Geometry check sheet. Reference: the model listing, model coordinates, mm. A direction names the side the tool comes from. Round coordinates to 2 decimals unless told otherwise and drop trailing zeros. Order: outer loops, then holes, each group sorted by start corner. A loop starts at its lowest first (then second) coordinate and runs counter-clockwise, first axis right, second up. Notation, with made-up numbers: (17, 31) -> (75, 31) arc R18 ccw to (75, 49) -> close; hole circle Ø4 at (19.5, 42). An arc over 180 degrees is marked (long way). Use a Markdown table: item, result. Add a question column.
Item 1: Gauge pin test, flat ends, axial feed: pin 1 Ø1 at (x, z) = (284.5, -15.5) entering from -Y; pin 2 Ø1.5 at (x, y) = (129, 3) entering from -Z; pin 3 Ø13 at (y, z) = (3, 1) entering from +X. Record the tip position at first contact, or that the pin passes through.
Item 2: Sectioned sample at A-A, the plane x = 343. Record the cut outline in (y, z), and give its area (3 significant figures).
Item 3: Material ranges on probe 1 along Z at (x, y) = (8.25, 0); probe 2 along Z at (x, y) = (312.5, -2); probe 3 along X at (y, z) = (16, -8.5), recorded low to high. Write a range as [from, to].
Item 4: Mould release check, pull along Y, two halves, no side actions. Record for faces 4 (the cylindrical face through (457.9, -14.18, 1.86)), 5 (the cylindrical face through (8.112, 2.285, 3.584)), 6 (the flat face through (12.4, 13, 0)): pulls with the +Y half, pulls with the -Y half, needs draft (parallel to the pull), parting line crosses it, or undercut.
Item 5: Set-up check for faces 1 (the flat face through (457.5, -11, -10)), 2 (the flat face through (13, -11, 10)), 3 (the cylindrical face through (232.18, -0.97, 22.06)): record each of +Z, -Z, +X, -X, +Y, -Y from which the full face is reachable in a straight line by a thin tool's end or side.
from build123d import *

# Parameters (mm, degrees)
F2_SIZE2 = 0.2309401077
F2_SIZE  = 0.4
F4_D     = 8.5


with BuildPart() as f1:
    # F0 (on Front) → F1 (revolve)
    with BuildSketch(Plane.XZ):
        with BuildLine():
            Line((0, 0), (0, -12.5))
            Line((0, -12.5), (12.4, -12.5))
            Line((12.4, -12.5), (12.4, -14.3))
            Line((12.4, -14.3), (12.8, -14.3))
            ThreePointArc((12.8, -14.3), (12.9414213562, -14.3585786438), (13, -14.5))
            Line((13, -14.5), (13, -23.582))
            ThreePointArc((13, -23.582), (13.4393398282, -24.6426601718), (14.5, -25.082))
            Line((14.5, -25.082), (456, -25.082))
            ThreePointArc((456, -25.082), (457.0606601718, -24.6426601718), (457.5, -23.582))
            Line((457.5, -23.582), (457.5, -14.5))
            ThreePointArc((457.5, -14.5), (457.5585786438, -14.3585786438), (457.7, -14.3))
            Line((457.7, -14.3), (458.1, -14.3))
            Line((458.1, -14.3), (458.1, -12.5))
            Line((458.1, -12.5), (470.5, -12.5))
            Line((470.5, -12.5), (470.5, -10.5))
            Line((470.5, -10.5), (454.5, -10.5))
            Line((454.5, -10.5), (454.5, -22.082))
            Line((454.5, -22.082), (16, -22.082))
            Line((16, -22.082), (16, 0))
            Line((16, 0), (0, 0))
        make_face()
    revolve(axis=Axis((8, 0, 0), (-1, 0, 0)))

    # F2
    f2_edges = [f1.edges().sort_by_distance(p)[0] for p in [
        (0, 0, 12.5),
    ]]
    f2_side = f1.faces().sort_by_distance((6.2, 0, 12.5))[0]
    chamfer(f2_edges, length=F2_SIZE, length2=F2_SIZE2, reference=f2_side)

    # F4 (through all)
    with Locations(Plane(origin=(0, 0, 0), x_dir=(0, -1, 0), z_dir=(-1, 0, 0))):
        with Locations((0, 0)):
            Hole(F4_D / 2)


solid = f1.part
Found:
| question | item | result |
|---|---|---|
| 1 | pin 1 | stops at y = -20.1 |
| 1 | pin 2 | stops at z = -24.98 |
| 1 | pin 3 | stops at x = 16 |
| 2 | outline | circle Ø50.16 at (0, 0); hole circle Ø44.16 at (0, 0) |
| 2 | area | 445 mm2 |
| 3 | probe 1 | z = [-12.5, -4.25], [4.25, 12.5] |
| 3 | probe 2 | z = [-25, -21.99], [21.99, 25] |
| 3 | probe 3 | x = [13, 16], [454.5, 457.5] |
| 4 | face 4 | parting line crosses it |
| 4 | face 5 | undercut |
| 4 | face 6 | needs draft |
| 5 | face 1 | +X |
| 5 | face 2 | -X |
| 5 | face 3 | none |
